Check sheet for the drawn part. Datum: minimum x, y, z corner. Units: mm. A direction names the side the tool comes from. Give positions to 0.01 mm unless a question says otherwise; leave off trailing zeros. Write each loop counter-clockwise with the first axis right and the second up, starting at its lowest first coordinate (ties: lowest second). Pieces come first, ordered by that corner, then holes. Notation, with made-up numbers: (-38.5, 79.25) -> (-9.5, 79.25) arc R19 ccw to (-9.5, 99.25) -> close; hole circle Ø2 at (58, 29.5). An arc over 180 degrees is marked (long way). Use CSV: the item, a comma, the result in double quotes. Start each with the question number.
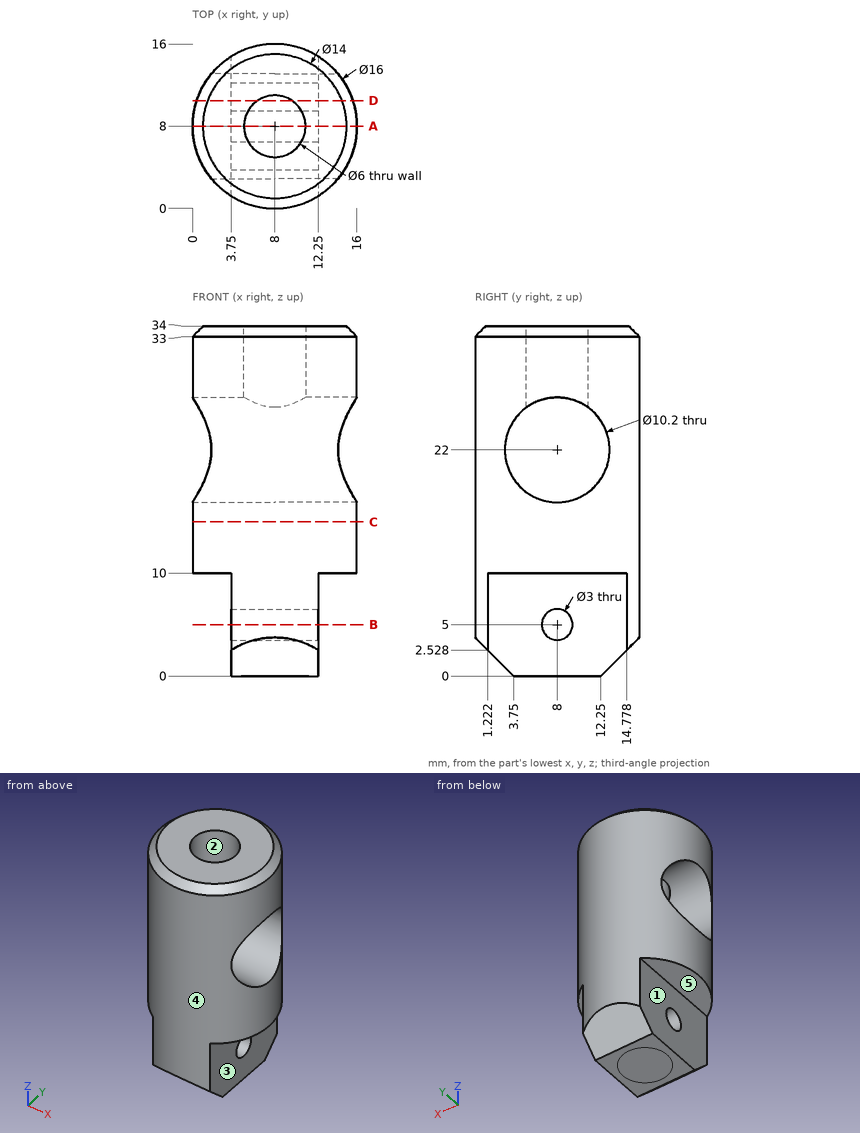
(1) Section check B-B on z = 5. Record the cut outline in (x, y), then the cut area to 3 significant figures.
(2) Section check A-A on y = 8. Record the cut outline in (x, z), then the cut area to 3 significant figures.
(3) Go/stop test with flat-tipped pins: pin 1 (3 mm diameter, centred on x = 2, y = 6.5, fed in from -Z); pin 2 (3.5 mm diameter, centred on y = 8, z = 5, fed in from +X); pin 3 (8 mm diameter, centred on y = 6, z = 21.5, fed in from -X). Record where each tip stops, or that it passes through.
(4) Section check C-C on z = 15. Record the cut outline in (x, y).
(5) Thickness scan on line 1 (Z direction, x = 9.25, y = 8); line 2 (Y direction, x = 8, z = 32.25); line 3 (Z direction, x = 11.75, y = 12) (1 decimal). Record the ranges inside material, lowest first. Write a range as from..to.
(6) Draft check along X on the marked faces 1, 2 and 3. Enter one of: released by +X, released by -X, zero draft, split by the parting line, or undercut.
(7) Set-up check for the marked faces 4 and 5: record each of +Z, -Z, +X, -X, +Y, -Y from which the full face is reachable in a straight line by a thin tool's end or side.
(8) Section check D-D on y = 10.5. Give the number of separate pieces and of enclosed holes in the cut face.
Data:
1,outline,"(3.75, 1.22) arc R8 ccw to (12.25, 1.22) -> (12.25, 6.5) -> (3.75, 6.5) -> close; (3.75, 9.5) -> (12.25, 9.5) -> (12.25, 14.78) arc R8 ccw to (3.75, 14.78) -> close"
1,area,"104 mm2"
2,outline,"(0, 10) -> (3.75, 10) -> (3.75, 6.5) -> (12.25, 6.5) -> (12.25, 10) -> (16, 10) -> (16, 16.9) -> (0, 16.9) -> close; (0, 27.1) -> (5, 27.1) -> (5, 34) -> (1, 34) -> (0, 33) -> close; (3.75, 0) -> (12.25, 0) -> (12.25, 3.5) -> (3.75, 3.5) -> close; (11, 27.1) -> (16, 27.1) -> (16, 33) -> (15, 34) -> (11, 34) -> close"
2,area,"238 mm2"
3,pin 1,"stops at z = 10"
3,pin 2,"stops at x = 12.25"
3,pin 3,"stops at x = 0.38"
4,outline,"circle Ø16 at (8, 8)"
5,line 1,"z = 0..3.5, 6.5..16.9"
5,line 2,"y = 0..5, 11..16"
5,line 3,"z = 0..18.8, 25.2..34"
6,face 1,"released by -X"
6,face 2,"undercut"
6,face 3,"released by +X"
7,face 4,"+Z, -Z"
7,face 5,"-Z, -X, +Y, -Y"
8,separate pieces,"3"
8,enclosed holes,"0"
